Here's the drawing with two shaded views (mm, measured from the low corner). I have some questions. A direction names the side the tool comes from. Round coordinates to 2 decimals unless told otherwise and drop trailing zeros. Loops run counter-clockwise (first coordinate to the right, second up) from the corner with the lowest first, then second, coordinate; pieces in that order, holes last.
(1) Which directions (+Z, -Z, +X, -X, +Y, -Y) give clear straight access to the entire face, cutting with the end or side of a thin tool? Please do the marked faces 5, 6, 7, 8 and 9.
(2) Thinking about a two-plate mould opening in X: for the marked faces 1, 2, 3 and 4, which applies, released by +X, released by -X, zero draft, split by the parting line, or undercut?
(3) Will these pins go through, and if not, where does the flat tip stop? pin 1 Ø1.5 at (y, z) = (6, 8.5) entering from -X; pin 2 Ø4 at (y, z) = (6, 3) entering from -X; pin 3 Ø5 at (x, y) = (11, 5.5) entering from -Z; pin 4 Ø1.9 at (y, z) = (4.5, 5) entering from +X.
(4) I want a section at C-C on x = 12. Write out the boundary of the cut face in (y, z), plus the area to 3 significant figures.
(5) I want a section at B-B on y = 4.5. Give the number of separate pieces and of enclosed holes in the cut face, plus the area to 3 significant figures.
(6) If I drill on line 1 along Y through (x, z) = (21, 12.35); line 2 along Z through (x, y) = (3.5, 2); line 3 along X through (y, z) = (4.25, 14.25), over which ranges is the centre line in solid material (lowest first)?
(7) I want a section at A-A on x = 4. Write out the boundary of the cut face in (y, z), plus the area to 3 significant figures.
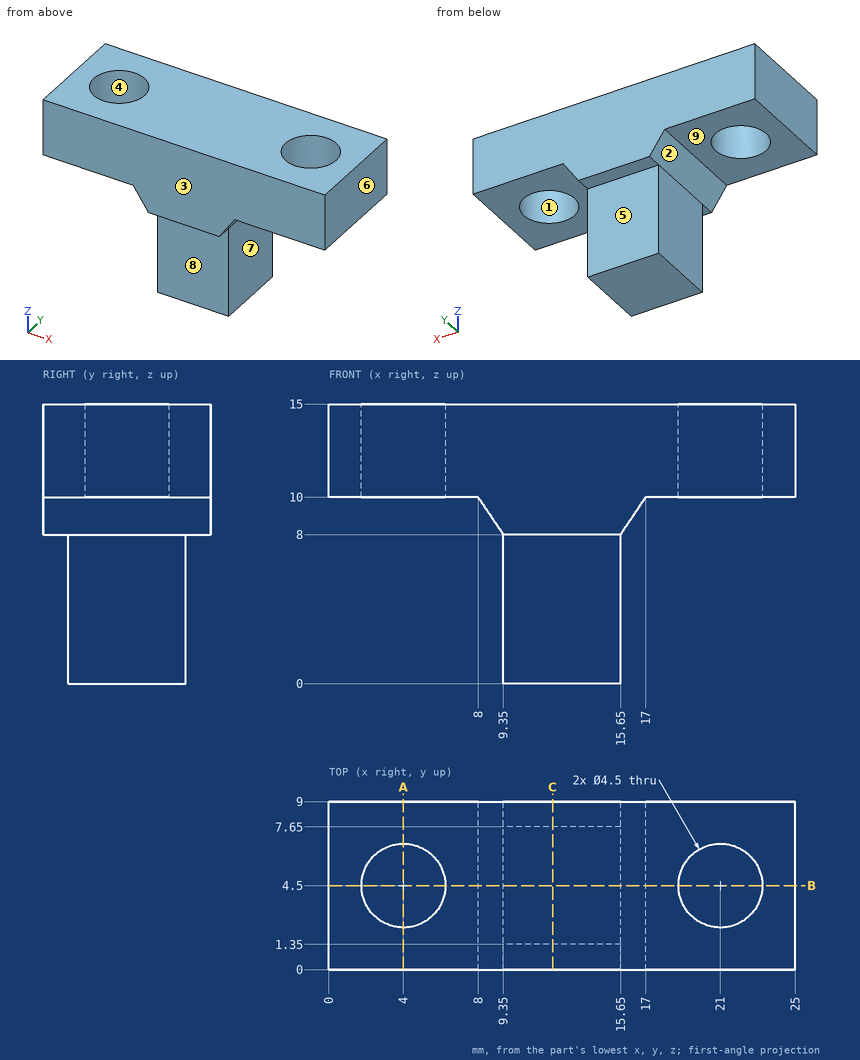
Filled sheet:
1. face 5: -Z, +X, -X, +Y
1. face 6: +Z, -Z, +X, +Y, -Y
1. face 7: -Z, +X, +Y, -Y
1. face 8: -Z, +X, -X, -Y
1. face 9: -Z, -X, +Y, -Y
2. face 1: undercut
2. face 2: released by -X
2. face 3: zero draft
2. face 4: undercut
3. pin 1: stops at x = 8.51
3. pin 2: stops at x = 9.35
3. pin 3: stops at z = 0
3. pin 4: stops at x = 15.65
4. outline: (0, 8) - (1.35, 8) - (1.35, 0) - (7.65, 0) - (7.65, 8) - (9, 8) - (9, 15) - (0, 15) - close
4. area: 113 mm2
5. separate pieces: 3
5. enclosed holes: 0
5. area: 146 mm2
6. line 1: y = 0 to 2.25, 6.75 to 9
6. line 2: z = 10 to 15
6. line 3: x = 0 to 1.76, 6.24 to 18.76, 23.24 to 25
7. outline: (0, 10) - (2.25, 10) - (2.25, 15) - (0, 15) - close; (6.75, 10) - (9, 10) - (9, 15) - (6.75, 15) - close
7. area: 22.5 mm2
